Can you work these out from the model? Positions are in its coordinate system, mm. Face numbers are marked on the shaded views. A direction names the side the tool comes from. Coordinates: 2 decimals unless noted, no trailing zeros. Order: outer loops, then holes, each group sorted by start corner. A loop starts at its lowest first (then second) coordinate and runs counter-clockwise, first axis right, second up. Notation, with made-up numbers: (-31.5, 53) - (18.5, 53) arc R37 ccw to (18.5, 91) - close; hole circle Ø6 at (42, 82.25). An arc over 180 degrees is marked (long way). Return JSON: item names as keys, results as strings. Group by question number.
1) Imagine slicing it at C-C (z = 22). Write out the boundary of the cut face in (x, y) (3 decimals).
2) If we mould it in two halves opening along Y, with no side actions, what happens to the marked faces 1, 2, 3 and 4? For each: pulls with the +Y half, pulls with the -Y half, needs draft (parallel to the pull), parting line crosses it, or undercut.
3) Which directions (+Z, -Z, +X, -X, +Y, -Y) give clear straight access to the entire face, cutting with the end or side of a thin tool? Please do the marked faces 5 and 6.
4) For pin 1 Ø4 at (x, z) = (-3, 10) entering from +Y; pin 2 Ø1.9 at (x, y) = (2.5, 1) entering from +Z; pin 3 Ø4 at (y, z) = (-3, -10) entering from +X, each with a flat end and sliding along its axis, tell me the tip position at first contact or that it passes through.
5) Imagine slicing it at D-D (y = -0.75). Write out the boundary of the cut face in (x, z).
6) If I drill on line 1 along X through (y, z) = (-2.5, -6); line 2 along Z through (x, y) = (-1.75, 2.5); line 3 along X through (y, z) = (2.75, -5.5), over which ranges is the centre line in solid material (lowest first)?
7) Imagine slicing it at B-B (z = 13). Write out the boundary of the cut face in (x, y).
8) Imagine slicing it at A-A (y = 1). Write out the boundary of the cut face in (x, z).
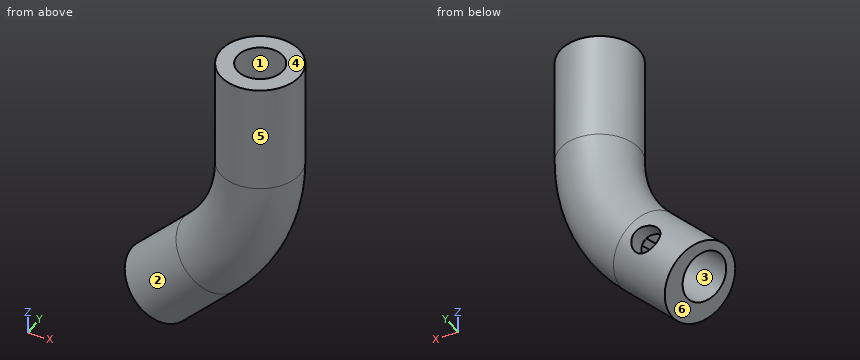
```python
from build123d import *

# Parameters (mm, degrees)
SKETCH4_R           = 5.5
SKETCH6_R           = 3.175
HOLE_SHAFT_DEPTH    = 10
SKETCH7_R           = 3.4
HOLE_POT_DEPTH      = 10
SKETCH8_R           = 2
HOLE_INSERT_DEPTH   = 6.5000001
BOSS_EXTRUDE3_DEPTH = 1.5


with BuildPart() as part:
    # Sweep2: sweep along a path in PROFILE
    with BuildLine(Plane(origin=(0, 0, 0), x_dir=(1, 0, 0), z_dir=(0, 1, 0))) as sweep2_path:
        Line((2.5, -25), (2.5, -10))
        ThreePointArc((2.5, -10), (0.747502348, -1.189599343), (-4.243188728, 6.27949768))
        Line((-4.243188728, 6.27949768), (-11.31425654, 13.350565492))
    # Sketch4 → Sweep2 (sweep)
    with BuildSketch(Plane.XY.offset(25)):
        with Locations((2.5, 0)):
            Circle(SKETCH4_R)
    sweep(path=sweep2_path.line)

    # Sketch6 → HOLE_SHAFT (cut)
    with BuildSketch(Plane.XY.offset(25)):
        with Locations((2.5, 0)):
            Circle(SKETCH6_R)
    extrude(amount=-HOLE_SHAFT_DEPTH, mode=Mode.SUBTRACT)

    # Sketch7 → HOLE_POT (cut)
    with BuildSketch(Plane(origin=(-12.332411016, 0, -12.332411016), x_dir=(-0.707106781, 0, 0.707106781), z_dir=(-0.707106781, 0, -0.707106781))):
        with Locations((-0.57444604, 0)):
            Circle(SKETCH7_R)
    extrude(amount=-HOLE_POT_DEPTH, mode=Mode.SUBTRACT)

    # Sketch8 → HOLE_INSERT (cut, through all)
    with BuildSketch(Plane(origin=(0, 0, 0), x_dir=(1, 0, 0), z_dir=(0, 1, 0))):
        with Locations((-6.673561157, 8.709870109)):
            Circle(SKETCH8_R)
    extrude(amount=HOLE_INSERT_DEPTH, mode=Mode.SUBTRACT)

    # Sketch11 → Boss-Extrude3 (add)
    with BuildSketch(Plane(origin=(-5.261343204, 0, -5.261343204), x_dir=(-0.707106781, 0, 0.707106781), z_dir=(-0.707106781, 0, -0.707106781))):
        with BuildLine():
            Line((-0.905457853, 3.383848575), (0.72667763, -3.141190411))
            ThreePointArc((0.72667763, -3.141190411), (0.250591719, -3.298380314), (-0.243434227, -3.383848575))
            Line((-0.243434227, -3.383848575), (-1.87556971, 3.141190411))
            ThreePointArc((-1.87556971, 3.141190411), (-1.3994838, 3.298380314), (-0.905457853, 3.383848575))
        make_face()
    extrude(amount=BOSS_EXTRUDE3_DEPTH)


solid = part.part
```
Calculated:
{
 "1": {"outline": "circle Ø11 at (2.5, 0); hole circle Ø6.35 at (2.5, 0)"},
 "2": {"face 1": "undercut", "face 2": "parting line crosses it", "face 3": "undercut", "face 4": "needs draft"},
 "3": {"face 5": "+Z", "face 6": "-Z, -X, +Y, -Y"},
 "4": {"pin 1": "y = 4.24", "pin 2": "z = 15", "pin 3": "x = 0.89"},
 "5": {"outline": "(-15.17, -9.5) - (-14.27, -10.39) - (-7.2, -3.32) - (-5.35, -5.17) - (-6.41, -6.23) - (-5.68, -6.96) - (-4.62, -5.9) - (-2.51, -8.01) - (-9.58, -15.08) - (-7.46, -17.2) - (-0.39, -10.13) arc R28.47 ccw to (7.95, 10) - (7.95, 25) - (5.59, 25) - (5.59, 15) - (-0.59, 15) - (-0.59, 25) - (-2.95, 25) - (-2.95, 10) arc R17.57 cw to (-8.1, -2.43) - close"},
 "6": {"line 1": "-10.89 to -8.45, -6.64 to -5.34, -4.52 to 2.36", "line 2": "-10.71 to 25", "line 3": "-10.2 to -7.52, -5.02 to 2.54"},
 "7": {"outline": "circle Ø11 at (2.5, 0)"},
 "8": {"outline": "(-15.14, -9.53) - (-14.22, -10.44) - (-7.15, -3.37) - (-5.04, -5.48) - (-6.1, -6.54) - (-5.37, -7.27) - (-4.31, -6.21) - (-2.56, -7.97) - (-9.63, -15.04) - (-7.49, -17.17) - (-0.42, -10.1) arc R28.43 ccw to (7.91, 10) - (7.91, 25) - (5.51, 25) - (5.51, 15) - (-0.51, 15) - (-0.51, 25) - (-2.91, 25) - (-2.91, 10) arc R17.61 cw to (-8.07, -2.46) - close"}
}
